Verification items for the finished model (mm, model axes). Face numbers are marked on the shaded views. A direction names the side the tool comes from. Give positions to 0.01 mm unless a question says otherwise; leave off trailing zeros. Loops run counter-clockwise (first coordinate to the right, second up) from the corner with the lowest first, then second, coordinate; pieces in that order, holes last. Notation, with made-up numbers: (40, 78.25) -> (55, 78.25) arc R31 cw to (55, 105.25) -> close; hole circle Ø3 at (15, -30.5). An arc over 180 degrees is marked (long way). Answer in a Markdown table with one row per item. Add a question column.
Q1. Set-up check for the marked faces 4, 5 and 6: record each of +Z, -Z, +X, -X, +Y, -Y from which the full face is reachable in a straight line by a thin tool's end or side.
Q2. Section check A-A on y = -3.75. Enter the section's corners in (x, z).
Q3. Section check B-B on z = -3. Enter the section's corners in (x, y), and give its area (3 significant figures).
Q4. Section check D-D on x = -0.5. Enter the section's corners in (y, z).
Q5. Release check for a two-part mould opening along X. For the marked faces 1, 2 and 3 record: pulls with the +X half, pulls with the -X half, needs draft (parallel to the pull), parting line crosses it, or undercut.
Q6. Material ranges on probe 1 along Z at (x, y) = (0, 1.4); probe 2 along Z at (x, y) = (-8.5, -0.25); probe 3 along X at (y, z) = (6.9, 15), recorded low to high.
Q7. Section check C-C on x = 8.5. Enter the section's corners in (y, z).
Q8. Gauge pin test, flat ends, axial feed: P1, Ø3.5, axis at x = 9, z = 13, coming from the -Y side; P2, Ø2, axis at x = -9, y = -9, coming from the -Z side; P3, Ø1.6, axis at x = -9.5, y = -9, coming from the +Z side. Record the tip position at first contact, or that the pin passes through.
```python
from build123d import *

# Parameters (mm, degrees)
SKETCH1_W           = 21
SKETCH1_H           = 50
SKETCH1_R           = 2.6
BOSS_EXTRUDE1_DEPTH = 8
SKETCH2_R           = 4.5
CUT_EXTRUDE1_DEPTH  = 5
SKETCH3_W           = 3
SKETCH3_H           = 10
BOSS_EXTRUDE2_DEPTH = 50
SKETCH4_W           = 2
SKETCH4_H           = 5
CUT_EXTRUDE2_DEPTH  = 22
FILLET1_R           = 5


with BuildPart() as part:
    # Sketch1 → Boss-Extrude1 (new body)
    with BuildSketch(Plane(origin=(0, 0, 0), x_dir=(1, 0, 0), z_dir=(0, 1, 0))):
        Rectangle(SKETCH1_W, SKETCH1_H)
        with Locations((0, -15)):
            Circle(SKETCH1_R, mode=Mode.SUBTRACT)
        with Locations((0, 15)):
            Circle(SKETCH1_R, mode=Mode.SUBTRACT)
    extrude(amount=BOSS_EXTRUDE1_DEPTH)

    # Sketch2 → Cut-Extrude1 (cut)
    with BuildSketch(Plane.XZ):
        with Locations((0, 15)):
            Circle(SKETCH2_R)
        with Locations((0, -15)):
            Circle(SKETCH2_R)
    extrude(amount=-CUT_EXTRUDE1_DEPTH, mode=Mode.SUBTRACT)

    # Sketch3 → Boss-Extrude2 (add)
    with BuildSketch(Plane.XY.offset(25)):
        with Locations((-9, -5)):
            Rectangle(SKETCH3_W, SKETCH3_H)
        with Locations((9, -5)):
            Rectangle(SKETCH3_W, SKETCH3_H)
    extrude(amount=-BOSS_EXTRUDE2_DEPTH)

    # Sketch4 → Cut-Extrude2 (cut, through all)
    with BuildSketch(Plane(origin=(10.5, 13.5, 0), x_dir=(0, -1, 0), z_dir=(1, 0, 0))):
        with Locations((14.5, -12.5)):
            Rectangle(SKETCH4_W, SKETCH4_H)
        with Locations((22.5, -12.5)):
            Rectangle(SKETCH4_W, SKETCH4_H)
        with Locations((22.5, 12.5)):
            Rectangle(SKETCH4_W, SKETCH4_H)
        with Locations((14.5, 12.5)):
            Rectangle(SKETCH4_W, SKETCH4_H)
    extrude(amount=-CUT_EXTRUDE2_DEPTH, mode=Mode.SUBTRACT)

    # Fillet1
    fillet1_edges = [part.edges().sort_by_distance(p)[0] for p in [
        (-9, -10, -25),
        (-9, -10, 25),
        (9, -10, 25),
        (9, -10, -25),
    ]]
    fillet(fillet1_edges, radius=FILLET1_R)


solid = part.part
```
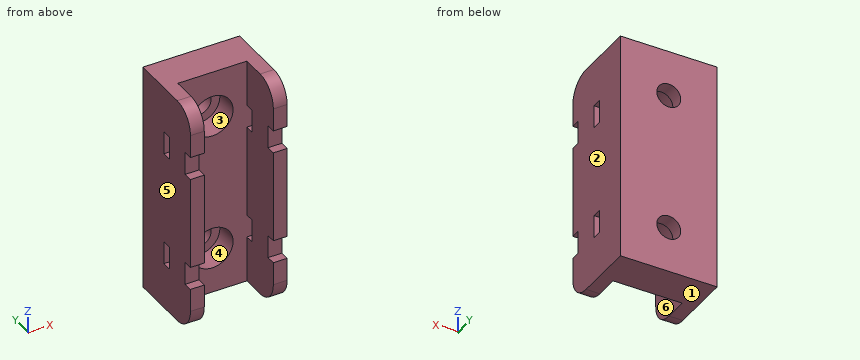
Taken from the geometry:
| question | item | result |
|---|---|---|
| 1 | face 4 | -Y |
| 1 | face 5 | +Z, -Z, -X, +Y, -Y |
| 1 | face 6 | +Z, -Z, -Y |
| 2 | outline | (-10.5, -25) -> (-7.5, -25) -> (-7.5, 25) -> (-10.5, 25) -> close; (7.5, -25) -> (10.5, -25) -> (10.5, 25) -> (7.5, 25) -> close |
| 3 | outline | (-10.5, -10) -> (-7.5, -10) -> (-7.5, 0) -> (7.5, 0) -> (7.5, -10) -> (10.5, -10) -> (10.5, 8) -> (-10.5, 8) -> close |
| 3 | area | 228 mm² |
| 4 | outline | (0, -25) -> (8, -25) -> (8, -17.55) -> (5, -17.55) -> (5, -19.47) -> (0, -19.47) -> close; (0, -10.53) -> (5, -10.53) -> (5, -12.45) -> (8, -12.45) -> (8, 12.45) -> (5, 12.45) -> (5, 10.53) -> (0, 10.53) -> close; (0, 19.47) -> (5, 19.47) -> (5, 17.55) -> (8, 17.55) -> (8, 25) -> (0, 25) -> close |
| 5 | face 1 | needs draft |
| 5 | face 2 | pulls with the +X half |
| 5 | face 3 | undercut |
| 6 | probe 1 | z = -25 to -19.5, -10.5 to 10.5, 19.5 to 25 |
| 6 | probe 2 | z = -25 to -15, -10 to 10, 15 to 25 |
| 6 | probe 3 | x = -10.5 to -2.6, 2.6 to 10.5 |
| 7 | outline | (-10, -20) arc R5 ccw to (-5, -25) -> (8, -25) -> (8, 25) -> (-5, 25) arc R5 ccw to (-10, 20) -> (-10, 15) -> (-8, 15) -> (-8, 10) -> (-10, 10) -> (-10, -10) -> (-8, -10) -> (-8, -15) -> (-10, -15) -> close; hole (-2, -15) -> (0, -15) -> (0, -10) -> (-2, -10) -> close; hole (-2, 10) -> (0, 10) -> (0, 15) -> (-2, 15) -> close |
| 8 | P1 | stops at y = -8 |
| 8 | P2 | stops at z = -24 |
| 8 | P3 | stops at z = 23.84 |
